Build history of the part. All positions in model axes, mm. Face numbers are marked on the shaded views. A direction names the side the tool comes from. Give positions to 0.01 mm unless a question says otherwise; leave off trailing zeros. Order: outer loops, then holes, each group sorted by start corner. A loop starts at its lowest first (then second) coordinate and runs counter-clockwise, first axis right, second up. Notation, with made-up numbers: (41.5, 69.25) - (97.5, 69.25) arc R16 cw to (97.5, 77.25) - close; hole circle Ø5 at (-30.5, 59.25). An arc over 180 degrees is marked (long way). One line per item, written item: value.
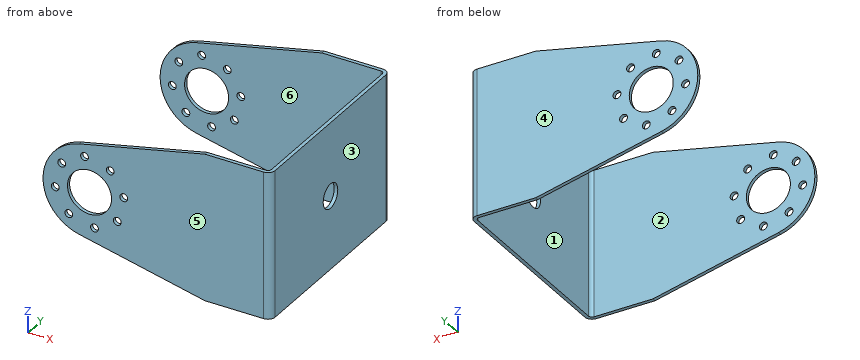
```python
from build123d import *

# Parameters (mm, degrees)
T_LE_DE_BASE_PLI_E1_DEPTH = 30
ESQUISSE13_R              = 4.5
ESQUISSE13_R_2            = 0.8
ENL_V_MAT_EXTRU_2_DEPTH   = 72.281133549
SKETCH1_R                 = 2.5
CUT_EXTRUDE1_DEPTH        = 60.052053397


# Sheet-metal steps are written as plain solids
with BuildPart() as part:
    # Esquisse1 → Tôle de base pliée1 (new body)
    with BuildSketch(Plane.XY):
        with BuildLine():
            Line((-50, 20.5), (-1.4732, 20.5))
            ThreePointArc((-1.4732, 20.5), (-0.43149029, 20.06850971), (0, 19.0268))
            Line((0, 19.0268), (0, -19.0268))
            ThreePointArc((0, -19.0268), (-0.43149029, -20.06850971), (-1.4732, -20.5))
            Line((-1.4732, -20.5), (-50, -20.5))
            Line((-50, -20.5), (-50, -19.7634))
            Line((-50, -19.7634), (-1.4732, -19.7634))
            ThreePointArc((-1.4732, -19.7634), (-0.952345145, -19.547654855), (-0.7366, -19.0268))
            Line((-0.7366, -19.0268), (-0.7366, 19.0268))
            ThreePointArc((-0.7366, 19.0268), (-0.952345145, 19.547654855), (-1.4732, 19.7634))
            Line((-1.4732, 19.7634), (-50, 19.7634))
            Line((-50, 19.7634), (-50, 20.5))
        make_face()
    extrude(amount=T_LE_DE_BASE_PLI_E1_DEPTH)

    # Esquisse13 → Enlèv. mat.-Extru.2 (cut, through all)
    with BuildSketch(Plane.XZ.offset(20.5)):
        with BuildLine():
            ThreePointArc((-46.549919552, 15), (-44.463516741, 20.940418901), (-39.120745506, 24.271552182))
            Line((-39.120745506, 24.271552182), (-13.4732, 30))
            Line((-13.4732, 30), (-50, 30))
            Line((-50, 30), (-50, 15))
            Line((-50, 15), (-46.549919552, 15))
        make_face()
        with BuildLine():
            Line((-13.4732, 0), (-39.120745506, 5.728447818))
            ThreePointArc((-39.120745506, 5.728447818), (-44.463516741, 9.059581099), (-46.549919552, 15))
            Line((-46.549919552, 15), (-50, 15))
            Line((-50, 15), (-50, 0))
            Line((-50, 0), (-13.4732, 0))
        make_face()
        with Locations((-37.049919552, 15)):
            Circle(ESQUISSE13_R)
        with Locations((-30.049919552, 16.017866465)):
            Circle(ESQUISSE13_R_2)
        with Locations((-32.819912364, 20.669487748)):
            Circle(ESQUISSE13_R_2)
        with Locations((-38.067786017, 22)):
            Circle(ESQUISSE13_R_2)
        with Locations((-42.7194073, 19.230007189)):
            Circle(ESQUISSE13_R_2)
        with Locations((-44.049919552, 13.982133535)):
            Circle(ESQUISSE13_R_2)
        with Locations((-41.279926741, 9.330512252)):
            Circle(ESQUISSE13_R_2)
        with Locations((-36.032053088, 8)):
            Circle(ESQUISSE13_R_2)
        with Locations((-31.380431805, 10.769992811)):
            Circle(ESQUISSE13_R_2)
    extrude(amount=-ENL_V_MAT_EXTRU_2_DEPTH, mode=Mode.SUBTRACT)

    # Sketch1 → Cut-Extrude1 (cut, through all)
    with BuildSketch(Plane(origin=(0, 0, 0), x_dir=(0, 0, -1), z_dir=(1, 0, 0))):
        with Locations(Location((-15, 0, 0), (0, 0, 90))):
            Circle(SKETCH1_R)
    extrude(amount=-CUT_EXTRUDE1_DEPTH, mode=Mode.SUBTRACT)


solid = part.part
```
(1) 3-axis set-ups, long thin cutter, end or side, ignore diameter. For the marked faces 5 and 6: which of +Z, -Z, +X, -X, +Y, -Y reach the whole face in a straight line?
Completed:
face 5: +Z, -Z, +X, -X, -Y
face 6: +Z, -Z, -X
(2) Slice it at B-B, the plane x = -3. Give the cut face in (y, z).
Completed:
outline: (-20.5, 0) - (-19.76, 0) - (-19.76, 30) - (-20.5, 30) - close; (19.76, 0) - (20.5, 0) - (20.5, 30) - (19.76, 30) - close
(3) Drill centre lines: line 1 (Y direction, x = -12.5, z = 18.5); line 2 (X direction, y = 13.5, z = 19). Where is each one in solid material? Low to high.
Completed:
line 1: -20.5 to -19.76, 19.76 to 20.5
line 2: -0.74 to 0
(4) Pin check, flat tip, straight feed: P1, Ø15, axis at y = -7.5, z = 22, coming from the -X side. Stop position of the tip, or through.
Completed:
P1: x = -0.74
(5) Slice it at A-A, the plane y = 0. Give the cut face in (x, z).
Completed:
outline: (-0.74, 0) - (0, 0) - (0, 12.5) - (-0.74, 12.5) - close; (-0.74, 17.5) - (0, 17.5) - (0, 30) - (-0.74, 30) - close
(6) Slice it at C-C, the plane z = 6.5. Give the cut face in (x, y), and give its area (3 significant figures).
Completed:
outline: (-41.29, -20.5) - (-1.47, -20.5) arc R1.47 ccw to (0, -19.03) - (0, 19.03) arc R1.47 ccw to (-1.47, 20.5) - (-41.29, 20.5) - (-41.29, 19.76) - (-1.47, 19.76) arc R0.74 cw to (-0.74, 19.03) - (-0.74, -19.03) arc R0.74 cw to (-1.47, -19.76) - (-41.29, -19.76) - close
area: 89.2 mm²
(7) Pull direction Y, two halves, no side cores. Call the marked faces 1, 2, 3 and 4: +Y half, -Y half, draft (parallel to the pull), parting line (faces both ways), or undercut.
Completed:
face 1: undercut
face 2: undercut
face 3: draft
face 4: +Y half
(8) Slice it at D-D, the plane y = -11.5. Give the cut face in (x, z), and give its area (3 significant figures).
Completed:
outline: (-0.74, 0) - (0, 0) - (0, 30) - (-0.74, 30) - close
area: 22.1 mm²
